Build history of the part. All positions in model axes, mm. A direction names the side the tool comes from. Give positions to 0.01 mm unless a question says otherwise; leave off trailing zeros. Loops run counter-clockwise (first coordinate to the right, second up) from the corner with the lowest first, then second, coordinate; pieces in that order, holes last. Notation, with made-up numbers: (66, 75.25) -> (75, 75.25) arc R10 cw to (75, 81.25) -> close; hole circle Ø8 at (86.25, -7). An arc over 180 degrees is marked (long way). Answer as a JSON object with one key per item and string values. Group by question number.
Q1. Band-saw the part on B-B, the plane x = 12. Write the cut outline in (y, z) (3 decimals).
Q2. Band-saw the part on C-C, the plane y = 0. Count the separate pieces of the cut face and the enclosed holes in it, plus the area to 3 significant figures.
Q3. Tool access for faces 1 (the flat face through (-4, 0, 33.655)), 2 (the flat face through (13.797, 0, 29)), 3 (the cylindrical face through (0.455, -3.463, 12.209)): list every direction of +Z, -Z, +X, -X, +Y, -Y with a clear straight run to the whole face (end or side of a thin tool).
Q4. Wall check: probe 1 along Z at (x, y) = (16, 6.25) (3 decimals); probe 2 along Y at (x, z) = (0, 7); probe 3 along X at (y, z) = (-1.25, 34). Give the ranges that are in metal, low to high. Write a range as from..to.
Q5. Two-plate mould, pull along Z, no slides. Class faces 4 (the flat face through (10, 0, 58.42)), 5 (the cylindrical face through (0.455, -3.463, 45.864)), 6 (the cylindrical face through (10.604, 4.606, 33.884)): pulls with the +Z half, pulls with the -Z half, needs draft (parallel to the pull), parting line crosses it, or undercut.
Q6. Drop flat-ended pins along their axis: pin 1 (7 mm diameter, centred on y = -1, z = 31, fed in from -X); pin 2 (6.5 mm diameter, centred on x = 0, y = 0, fed in from +Z); pin 3 (1.8 mm diameter, centred on y = 4.34, z = 32.9, fed in from -X); pin 4 (3 mm diameter, centred on y = -2.5, z = 31, fed in from +X). Give the stop position or say it passes through.
Q7. Band-saw the part on A-A, the plane z = 40. Write the cut outline in (x, y) (1 decimal), plus the area to 3 significant figures.
from build123d import *

# Parameters (mm, degrees)
SKETCH1_R           = 3.4925
BOSS_EXTRUDE1_DEPTH = 58.42
SKETCH2_W           = 21.884407041
SKETCH2_H           = 12.7
SKETCH2_W_2         = 26.524954362
SKETCH2_W_3         = 12.7
SKETCH2_H_2         = 8.89
CUT_EXTRUDE1_DEPTH  = 14.224
SKETCH4_W           = 15.997333927
SKETCH4_H           = 8.89
CUT_EXTRUDE2_DEPTH  = 14.224
SKETCH5_R           = 0.7366
SKETCH5_R_2         = 1.016
CUT_EXTRUDE3_DEPTH  = 12.7


with BuildPart() as part:
    # Sketch1 → Boss-Extrude1 (new body)
    with BuildSketch(Plane.XY):
        with BuildLine():
            Line((0, 7.112), (19.05, 7.112))
            ThreePointArc((19.05, 7.112), (26.162, 0), (19.05, -7.112))
            Line((19.05, -7.112), (0, -7.112))
            ThreePointArc((0, -7.112), (-7.112, 0), (0, 7.112))
        make_face()
        with Locations(Location((0, 0, 0), (0, 0, 180))):
            Circle(SKETCH1_R, mode=Mode.SUBTRACT)
        with Locations(Location((19.05, 0, 0), (0, 0, 180))):
            Circle(SKETCH1_R, mode=Mode.SUBTRACT)
    extrude(amount=BOSS_EXTRUDE1_DEPTH)

    # Sketch2 → Cut-Extrude1 (cut)
    with BuildSketch(Plane(origin=(0, 7.112, 0), x_dir=(1, 0, 0), z_dir=(0, 1, 0))):
        with Locations((22.372203521, -13.97)):
            Rectangle(SKETCH2_W, SKETCH2_H)
        with Locations((24.692477181, -44.45)):
            Rectangle(SKETCH2_W_2, SKETCH2_H)
        with Locations((20.147317334, -29.21)):
            Rectangle(SKETCH2_W_3, SKETCH2_H_2)
    extrude(amount=-CUT_EXTRUDE1_DEPTH, mode=Mode.SUBTRACT)

    # Sketch4 → Cut-Extrude2 (cut)
    with BuildSketch(Plane(origin=(0, 7.112, 0), x_dir=(1, 0, 0), z_dir=(0, 1, 0))):
        with Locations((-2.244730027, -29.21)):
            Rectangle(SKETCH4_W, SKETCH4_H)
    extrude(amount=-CUT_EXTRUDE2_DEPTH, mode=Mode.SUBTRACT)

    # Sketch5 → Cut-Extrude3 (cut)
    with BuildSketch(Plane.ZY.offset(-5.753936937)):
        with Locations((25.537266397, 4.339945309)):
            Circle(SKETCH5_R)
        with Locations(Location((32.903266397, 4.339945309, 0), (0, 0, 317.722495694))):
            Circle(SKETCH5_R_2)
    extrude(amount=-CUT_EXTRUDE3_DEPTH, mode=Mode.SUBTRACT)


solid = part.part
Worked answers:
{
 "1": {"outline": "(-7.112, 0) -> (7.112, 0) -> (7.112, 7.62) -> (-7.112, 7.62) -> close; (-7.112, 20.32) -> (7.112, 20.32) -> (7.112, 38.1) -> (-7.112, 38.1) -> close; (-7.112, 50.8) -> (7.112, 50.8) -> (7.112, 58.42) -> (-7.112, 58.42) -> close; hole circle Ø2.032 at (4.34, 32.903); hole circle Ø1.473 at (4.34, 25.537)"},
 "2": {"separate pieces": "7", "enclosed holes": "0", "area": "831 mm2"},
 "3": {"face 1": "-X, +Y, -Y", "face 2": "+X, +Y, -Y", "face 3": "+Z, -Z"},
 "4": {"probe 1": "0..7.62, 20.32..24.765, 33.655..38.1, 50.8..58.42", "probe 2": "-7.11..-3.49, 3.49..7.11", "probe 3": "-7..-3.26, 3.26..15.79, 22.31..26.05"},
 "5": {"face 4": "pulls with the +Z half", "face 5": "needs draft", "face 6": "undercut"},
 "6": {"pin 1": "x = -7.11", "pin 2": "through", "pin 3": "x = -5.98", "pin 4": "x = 13.8"},
 "7": {"outline": "(0, -7.1) -> (11.4, -7.1) -> (11.4, 7.1) -> (0, 7.1) arc R7.1 ccw to start; hole circle Ø7 at (0, 0)", "area": "204 mm2"}
}
